Geometry check sheet. Reference: the model listing, model coordinates, mm. A direction names the side the tool comes from. Coordinates: 2 decimals unless noted, no trailing zeros. Answer in a Markdown table with one row per item. Add a question column.
Q1. Gauge pin test, flat ends, axial feed: P1, Ø10, axis at x = 59, y = 70.5, coming from the -Z side; P2, Ø1, axis at x = 48, z = -2.5, coming from the +Y side; P3, Ø3, axis at x = 37, z = -2.5, coming from the -Y side. Record the tip position at first contact, or that the pin passes through.
Q2. Tool access check on faces 5 (the face through (76, 0, 0)), 6 (the face through (12.2, 27.2, -0.4)), 7 (the face through (69.85, 16, 0)). Record the directions out of +Z, -Z, +X, -X, +Y, -Y that give a thin tool (end or side, any length) a straight path to the whole face; none if there is none.
Q3. Release check for a two-part mould opening along X. For faces 1 (the face through (32, 53, 4.762)), 2 (the face through (14.388, 19, -1)), 3 (the face through (51, 32.512, 0)), 4 (the face through (82.55, 25, 0)) record: pulls with the +X half, pulls with the -X half, needs draft (parallel to the pull), parting line crosses it, or undercut.
Q4. Thickness scan on line 1 (X direction, y = 17.5, z = 2.25); line 2 (X direction, y = 30, z = 0.25); line 3 (Y direction, x = 22, z = 2.5). Record the ranges inside material, lowest first.
```python
from build123d import *

# Parameters (mm, degrees)
CORE_DEPTH                = 4.7625
CORE_DEPTH_BACK           = 4.7625
LEADINGEDGE_START         = -118.279773997
LEADINGEDGE_DEPTH         = 144.703179824
CTRLSURFCUTOUT_DEPTH      = 174.386689122
CTRLSURFCUTOUT_DEPTH_BACK = 174.386689122
SERVOPKT_DEPTH            = 8.516499985
WIREPKT_START             = -8.516499985
WIREPKT_DEPTH             = 8.516499985


# Read off the part's stored shape, not the designer's step: LeadingEdge, WirePkt
with BuildPart() as part:
    # Sketch2 → Core (new, two sides: drawn at the far end of the back side and taken through both)
    with BuildSketch(Plane.XY.offset(-CORE_DEPTH_BACK)):
        Polygon((0, 0), (82.55, 0), (82.55, 50.8), (0, 152.4), align=None)
    extrude(amount=CORE_DEPTH + CORE_DEPTH_BACK)

    # LeadingEdge outline → LeadingEdge (cut)
    with BuildSketch(Plane(origin=(0, 0, 0), x_dir=(0.7761140001162661, 0.630592625094465, 0), z_dir=(0.6305926250944651, -0.776114000116266, 0)).offset(LEADINGEDGE_START)):
        with BuildLine():
            Line((96.102316064, 4.7625), (84.894223283, 4.7625))
            add(Edge.make_bspline(
                [(84.894223283, 4.7625), (91.459772026, 4.7625), (96.102316064, 2.789807909), (96.102316064, 0)],
                knots=[0, 0, 0, 0, 1, 1, 1, 1], degree=3, weights=[1, 0.804737854, 0.804737854, 1]))
            Line((96.102316064, 0), (96.102316064, 4.7625))
        make_face()
    leadingedge = extrude(amount=LEADINGEDGE_DEPTH, mode=Mode.SUBTRACT)

    # LeadingEdgeMirror: LeadingEdge across plane
    add(leadingedge.mirror(Plane.XY), mode=Mode.SUBTRACT)

    # Sketch4 → CtrlSurfCutout (cut, two sides: drawn at the far end of the back side and taken through both)
    with BuildSketch(Plane.XY.offset(-CTRLSURFCUTOUT_DEPTH_BACK)):
        Polygon((31.242, 0), (69.85, 0), (69.85, 31.75), (69.85, 32.512), (69.596, 32.512), (31.496, 32.512), (31.242, 32.512), align=None)
    extrude(amount=CTRLSURFCUTOUT_DEPTH + CTRLSURFCUTOUT_DEPTH_BACK, mode=Mode.SUBTRACT)

    # Sketch7 → ServoPkt (cut)
    with BuildSketch(Plane(origin=(0, 0, -4.7625), x_dir=(-1, 0, 0), z_dir=(0, 0, -1))):
        with BuildLine():
            Line((-31.242, 32.241499906), (-17.562999926, 32.241499906))
            ThreePointArc((-17.562999926, 32.241499906), (-15.317935896, 31.311563936), (-14.387999926, 29.066499906))
            Line((-14.387999926, 29.066499906), (-14.387999926, 11.733500028))
            ThreePointArc((-14.387999926, 11.733500028), (-17.562999926, 8.558500028), (-20.737999926, 11.733500028))
            Line((-20.737999926, 11.733500028), (-31.242, 11.733500028))
            Line((-31.242, 11.733500028), (-31.242, 32.241499906))
        make_face()
    extrude(amount=-SERVOPKT_DEPTH, mode=Mode.SUBTRACT)

    # WirePkt outline → WirePkt (cut)
    with BuildSketch(Plane(origin=(0, 0, -4.7625), x_dir=(-1, 0, 0), z_dir=(0, 0, -1)).offset(WIREPKT_START)):
        with BuildLine():
            Line((-14.387999926, 29.066499906), (-14.387999926, 26.261862953))
            ThreePointArc((-14.387999926, 26.261862953), (-12.181797279, 27.210752433), (-10.283063956, 28.681307815))
            Line((-10.283063956, 28.681307815), (0, 38.964371771))
            Line((0, 38.964371771), (0, 47.944627893))
            Line((0, 47.944627893), (-14.773192017, 33.171435876))
            ThreePointArc((-14.773192017, 33.171435876), (-15.803236149, 32.48318239), (-17.018256047, 32.241499906))
            Line((-17.018256047, 32.241499906), (-17.562999926, 32.241499906))
            ThreePointArc((-17.562999926, 32.241499906), (-15.317935896, 31.311563936), (-14.387999926, 29.066499906))
        make_face()
    extrude(amount=WIREPKT_DEPTH, mode=Mode.SUBTRACT)


solid = part.part
```
Calculated:
| question | item | result |
|---|---|---|
| 1 | P1 | stops at z = -4.76 |
| 1 | P2 | stops at y = 91.87 |
| 1 | P3 | stops at y = 32.51 |
| 2 | face 5 | +Z, -Z, +X, -X, -Y |
| 2 | face 6 | -Z |
| 2 | face 7 | +Z, -Z, -Y |
| 3 | face 1 | needs draft |
| 3 | face 2 | undercut |
| 3 | face 3 | undercut |
| 3 | face 4 | pulls with the +X half |
| 4 | line 1 | x = 0 to 14.39, 69.85 to 82.55 |
| 4 | line 2 | x = 0 to 8.96, 69.85 to 82.55 |
| 4 | line 3 | y = 0 to 11.73, 32.24 to 122.68 |
